from build123d import *

# Parameters (mm, degrees)
SKETCH1_W           = 7.8
SKETCH1_H           = 7.3
SKETCH1_R           = 2
SKETCH1_W_2         = 8.2
SKETCH1_H_2         = 8
SKETCH1_H_3         = 6.8
SKETCH1_W_3         = 8.1
BOSS_EXTRUDE1_DEPTH = 8


with BuildPart() as part:
    # Sketch1 → Boss-Extrude1 (new body)
    # profile 1 of 5: a face of its own
    with BuildSketch(Plane.XY):
        with Locations((-31.25, 56.65)):
            Rectangle(SKETCH1_W, SKETCH1_H)
        with Locations((-31.25, 56.65)):
            Circle(SKETCH1_R, mode=Mode.SUBTRACT)
    # profile 2 of 5: a face of its own
    with BuildSketch(Plane.XY):
        Polygon((-27.35, 53), (-35.15, 53), (-35.15, -53), (-26.95, -53), (27.05, -53), (35.15, -53), (35.15, 53), (26.95, 53), align=None)
    # profile 3 of 5: a face of its own
    with BuildSketch(Plane.XY):
        with Locations((-31.05, -57)):
            Rectangle(SKETCH1_W_2, SKETCH1_H_2)
        with Locations((-31.05, -57)):
            Circle(SKETCH1_R, mode=Mode.SUBTRACT)
    # profile 4 of 5: a face of its own
    with BuildSketch(Plane.XY):
        with Locations((31.05, 56.4)):
            Rectangle(SKETCH1_W_2, SKETCH1_H_3)
        with Locations((31.05, 56.4)):
            Circle(SKETCH1_R, mode=Mode.SUBTRACT)
    # profile 5 of 5: a face of its own
    with BuildSketch(Plane.XY):
        with Locations((31.1, -57)):
            Rectangle(SKETCH1_W_3, SKETCH1_H_2)
        with Locations((31.1, -57)):
            Circle(SKETCH1_R, mode=Mode.SUBTRACT)
    extrude(amount=BOSS_EXTRUDE1_DEPTH)


solid = part.part
Verification items for the finished model (mm, model axes). A direction names the side the tool comes from. Give positions to 0.01 mm unless a question says otherwise; leave off trailing zeros. Write each loop counter-clockwise with the first axis right and the second up, starting at its lowest first coordinate (ties: lowest second). Pieces come first, ordered by that corner, then holes. Notation, with made-up numbers: (-31.75, 87.25) - (-7.75, 87.25) arc R21 cw to (-7.75, 105.25) - close; hole circle Ø8 at (64.5, 34). An arc over 180 degrees is marked (long way). Answer as CSV lines item,"result". Start each with the question number.
1. Sectioned sample at D-D (x = -4). Record the boundary of the cut face in (y, z), then the cut area to 3 significant figures.
2. Sectioned sample at B-B (x = -31.25). Record the boundary of the cut face in (y, z).
3. Sectioned sample at A-A (y = -57). Record the boundary of the cut face in (x, z), then the cut area to 3 significant figures.
4. Sectioned sample at C-C (z = 6.5). Record the boundary of the cut face in (x, y), then the cut area to 3 significant figures.
5. Set-up check for faces 4 (the face through (31, 59.8, 4)), 5 (the face through (31, -61, 4)), 6 (the face through (26.95, 56, 4)), 7 (the face through (-26.95, -57, 4)): record each of +Z, -Z, +X, -X, +Y, -Y from which the full face is reachable in a straight line by a thin tool's end or side.
6. Thickness scan on line 1 (Y direction, x = 31.05, z = 4.25); line 2 (Y direction, x = -31.05, z = 4.5); line 3 (Y direction, x = 25.5, z = 6.25). Record the ranges inside material, lowest first.
7. Draft check along X on faces 1 (the face through (-35.15, 0, 4)), 2 (the face through (27.05, -57, 4)), 3 (the face through (-31, 60.3, 4)). Enter one of: pulls with the +X half, pulls with the -X half, needs draft (parallel to the pull), parting line crosses it, or undercut.
8. Depth check by flat-ended pin: pin 1 (3 mm diameter, centred on x = 31.1, y = -57, fed in from -Z); pin 2 (1 mm diameter, centred on x = 24.5, z = 6.5, fed in from -Y); pin 3 (2.5 mm diameter, centred on x = 30, z = 3, fed in from +Y); pin 4 (1.5 mm diameter, centred on x = 7, z = 5.5, fed in from +Y). Enter the tip coordinate at first touch or a pass-through.
Derived:
1,outline,"(-53, 0) - (53, 0) - (53, 8) - (-53, 8) - close"
1,area,"848 mm²"
2,outline,"(-61, 0) - (-58.99, 0) - (-58.99, 8) - (-61, 8) - close; (-55.01, 0) - (54.65, 0) - (54.65, 8) - (-55.01, 8) - close; (58.65, 0) - (60.3, 0) - (60.3, 8) - (58.65, 8) - close"
3,outline,"(-35.15, 0) - (-33.05, 0) - (-33.05, 8) - (-35.15, 8) - close; (-29.05, 0) - (-26.95, 0) - (-26.95, 8) - (-29.05, 8) - close; (27.05, 0) - (29.1, 0) - (29.1, 8) - (27.05, 8) - close; (33.1, 0) - (35.15, 0) - (35.15, 8) - (33.1, 8) - close"
3,area,"66.4 mm²"
4,outline,"(-35.15, -61) - (-26.95, -61) - (-26.95, -53) - (27.05, -53) - (27.05, -61) - (35.15, -61) - (35.15, 59.8) - (26.95, 59.8) - (26.95, 53) - (-27.35, 53) - (-27.35, 60.3) - (-35.15, 60.3) - close; hole circle Ø4 at (-31.25, 56.65); hole circle Ø4 at (-31.05, -57); hole circle Ø4 at (31.05, 56.4); hole circle Ø4 at (31.1, -57)"
4,area,"7,640 mm²"
5,face 4,"+Z, -Z, +X, +Y"
5,face 5,"+Z, -Z, +X, -X, -Y"
5,face 6,"+Z, -Z, +Y"
5,face 7,"+Z, -Z, -Y"
6,line 1,"-61 to -59, -55 to 54.4, 58.4 to 59.8"
6,line 2,"-61 to -59, -55 to 54.66, 58.64 to 60.3"
6,line 3,"-53 to 53"
7,face 1,"pulls with the -X half"
7,face 2,"undercut"
7,face 3,"needs draft"
8,pin 1,"through"
8,pin 2,"y = -53"
8,pin 3,"y = 59.8"
8,pin 4,"y = 53"
